from build123d import *

# Parameters (mm, degrees)
F1_W     = 200
F1_H     = 10.5
F1_R     = 1.75
F2_DEPTH = 1.6
F3_R     = 1.75


# Not quite as in the source:
# - a fillet or chamfer that OpenCascade refuses, or shapes differently, is made with other operations: its cross-section is extruded or revolved along the edge and cut away or added
# - a feature names something its author has since deleted; it is built from what else it names


with BuildPart() as f2:
    # F1 (on Top) → F2 (new body)
    with BuildSketch(Plane.XY):
        with Locations((100, 5.25)):
            Rectangle(F1_W, F1_H)
        with BuildLine():
            ThreePointArc((78, 7), (79.75, 5.25), (78, 3.5))
            Line((78, 3.5), (5.25, 3.5))
            ThreePointArc((5.25, 3.5), (3.5, 5.25), (5.25, 7))
            Line((5.25, 7), (78, 7))
        make_face(mode=Mode.SUBTRACT)
        with Locations((85, 5.25)):
            Circle(F1_R, mode=Mode.SUBTRACT)
        with Locations((115, 5.25)):
            Circle(F1_R, mode=Mode.SUBTRACT)
        with BuildLine():
            Line((122, 7), (194.75, 7))
            ThreePointArc((194.75, 7), (196.5, 5.25), (194.75, 3.5))
            Line((194.75, 3.5), (122, 3.5))
            ThreePointArc((122, 3.5), (120.25, 5.25), (122, 7))
        make_face(mode=Mode.SUBTRACT)
    extrude(amount=F2_DEPTH)

    # F3
    f3_edges = [f2.edges().sort_by_distance(p)[0] for p in [
        (0, 10.5, 0.8),
        (0, 0, 0.8),
        (200, 0, 0.8),
        (200, 10.5, 0.8),
    ]]
    fillet(f3_edges, radius=F3_R)

    # F4: chamfer of 1.75 on 2 edges, made by hand

    # F4_s1 → F4_t2 (revolve, cut)
    with BuildSketch(Plane.XZ.offset(-5.25)):
        Polygon((88.5, 1.6), (86.75, -0.15), (86.75, 1.6), align=None)
    revolve(axis=Axis((85, 5.25, 1.6), (0, 0, 1)), mode=Mode.SUBTRACT)

    # F4_s3 → F4_t4 (revolve, cut)
    with BuildSketch(Plane.XZ.offset(-5.25)):
        Polygon((118.5, 1.6), (116.75, -0.15), (116.75, 1.6), align=None)
    revolve(axis=Axis((115, 5.25, 1.6), (0, 0, 1)), mode=Mode.SUBTRACT)


solid = f2.part
Input: part model. Units: mm. Frame: model coordinates. Give positions to 0.01 mm unless a question says otherwise; leave off trailing zeros. Order: outer loops, then holes, each group sorted by start corner. A loop starts at its lowest first (then second) coordinate and runs counter-clockwise, first axis right, second up. Notation, with made-up numbers: M -20.75,-37 L 12.25,-37 A26 cw 12.25,0 Z; hole C -19,11.5 d1. An arc over 180 degrees is marked long. Answer as a JSON object with one key per item and string values.
1. Cut plane C-C, the plane x = 161. Output: boundary loops of the cut face in (y, z), and give its area (3 significant figures).
Result sheet:
{"outline": "M 0,0 L 3.5,0 L 3.5,1.6 L 0,1.6 Z; M 7,0 L 10.5,0 L 10.5,1.6 L 7,1.6 Z", "area": "11.2 mm²"}
2. Cut plane D-D, the plane x = 85. Output: boundary loops of the cut face in (y, z).
Result sheet:
{"outline": "M 0,0 L 3.35,0 L 1.75,1.6 L 0,1.6 Z; M 7.15,0 L 10.5,0 L 10.5,1.6 L 8.75,1.6 Z"}
3. Ray query, line 1 (Y direction, x = 178.5, z = 0.95); line 2 (X direction, y = 4.25, z = 0.85); line 3 (X direction, y = 7.5, z = 0.65). Return the intervals inside material, ascending. Write a range as [from, to].
Result sheet:
{"line 1": "[0, 3.5], [7, 10.5]", "line 2": "[0, 3.81], [79.44, 82.44], [87.56, 112.44], [117.56, 120.56], [196.19, 200]", "line 3": "[0, 83.8], [86.2, 113.8], [116.2, 200]"}
4. Cut plane A-A, the plane y = 5.25. Output: boundary loops of the cut face in (x, z).
Result sheet:
{"outline": "M 0,0 L 3.5,0 L 3.5,1.6 L 0,1.6 Z; M 79.75,0 L 83.1,0 L 81.5,1.6 L 79.75,1.6 Z; M 86.9,0 L 113.1,0 L 111.5,1.6 L 88.5,1.6 Z; M 116.9,0 L 120.25,0 L 120.25,1.6 L 118.5,1.6 Z; M 196.5,0 L 200,0 L 200,1.6 L 196.5,1.6 Z"}
5. Cut plane B-B, the plane z = 0.55. Output: boundary loops of the cut face in (x, y), and give its area (3 significant figures).
Result sheet:
{"outline": "M 0,1.75 A1.75 ccw 1.75,0 L 198.25,0 A1.75 ccw 200,1.75 L 200,8.75 A1.75 ccw 198.25,10.5 L 1.75,10.5 A1.75 ccw 0,8.75 Z; hole M 5.25,3.5 L 78,3.5 A1.75 ccw 78,7 L 5.25,7 A1.75 ccw Z; hole C 85,5.25 d4.9; hole C 115,5.25 d4.9; hole M 122,3.5 L 194.75,3.5 A1.75 ccw 194.75,7 L 122,7 A1.75 ccw Z", "area": "1,530 mm²"}
